from build123d import *

# Parameters (mm, degrees)
SKETCH1_W           = 68
SKETCH1_H           = 33
SKETCH1_R           = 0.95
SKETCH1_W_2         = 52
SKETCH1_H_2         = 17
BOSS_EXTRUDE1_DEPTH = 2
SKETCH2_R           = 4
SKETCH2_R_2         = 0.95
BOSS_EXTRUDE2_DEPTH = 6
FILLET1_R           = 5


with BuildPart() as part:
    # Sketch1 → Boss-Extrude1 (new body)
    with BuildSketch(Plane.XY):
        Rectangle(SKETCH1_W, SKETCH1_H)
        with Locations((-29, 11.5)):
            Circle(SKETCH1_R, mode=Mode.SUBTRACT)
        with Locations((29, 11.5)):
            Circle(SKETCH1_R, mode=Mode.SUBTRACT)
        with Locations((29, -11.5)):
            Circle(SKETCH1_R, mode=Mode.SUBTRACT)
        with Locations((-29, -11.5)):
            Circle(SKETCH1_R, mode=Mode.SUBTRACT)
        Rectangle(SKETCH1_W_2, SKETCH1_H_2, mode=Mode.SUBTRACT)
    extrude(amount=BOSS_EXTRUDE1_DEPTH)

    # Sketch2 → Boss-Extrude2 (add)
    # profile 1 of 4: a face of its own
    with BuildSketch(Plane.XY.offset(2)):
        with Locations(Location((-29, 11.5, 0), (0, 0, 180))):
            Circle(SKETCH2_R)
        with Locations((-29, 11.5)):
            Circle(SKETCH2_R_2, mode=Mode.SUBTRACT)
    # profile 2 of 4: a face of its own
    with BuildSketch(Plane.XY.offset(2)):
        with Locations(Location((29, 11.5, 0), (0, 0, 180))):
            Circle(SKETCH2_R)
        with Locations((29, 11.5)):
            Circle(SKETCH2_R_2, mode=Mode.SUBTRACT)
    # profile 3 of 4: a face of its own
    with BuildSketch(Plane.XY.offset(2)):
        with Locations(Location((29, -11.5, 0), (0, 0, 180))):
            Circle(SKETCH2_R)
        with Locations((29, -11.5)):
            Circle(SKETCH2_R_2, mode=Mode.SUBTRACT)
    # profile 4 of 4: a face of its own
    with BuildSketch(Plane.XY.offset(2)):
        with Locations(Location((-29, -11.5, 0), (0, 0, 180))):
            Circle(SKETCH2_R)
        with Locations((-29, -11.5)):
            Circle(SKETCH2_R_2, mode=Mode.SUBTRACT)
    extrude(amount=BOSS_EXTRUDE2_DEPTH)

    # Fillet1
    fillet1_edges = [part.edges().sort_by_distance(p)[0] for p in [
        (26, -8.5, 1),
        (26, 8.5, 1),
        (-26, 8.5, 1),
        (-26, -8.5, 1),
        (34, -16.5, 1),
        (-34, -16.5, 1),
        (-34, 16.5, 1),
        (34, 16.5, 1),
    ]]
    fillet(fillet1_edges, radius=FILLET1_R)


solid = part.part
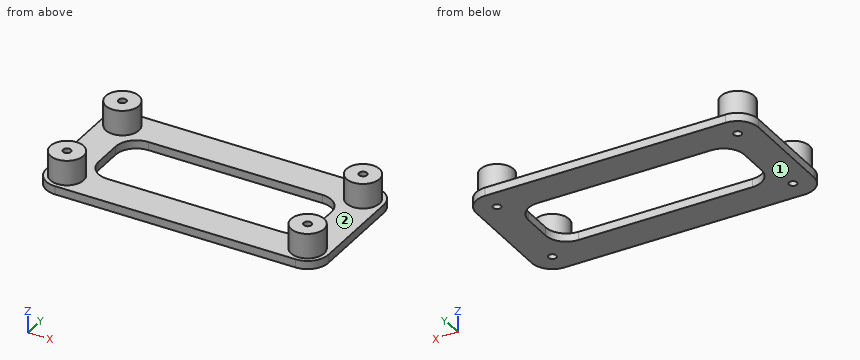
Geometry check sheet. Reference: the model listing, model coordinates, mm. Face numbers are marked on the shaded views. Give positions to 0.01 mm unless a question says otherwise; leave off trailing zeros. Write each loop counter-clockwise with the first axis right and the second up, starting at its lowest first coordinate (ties: lowest second). Pieces come first, ordered by that corner, then holes. Notation, with made-up numbers: M 53.25,-39 L 67.25,-39 A27 ccw 67.25,-22 Z; hole C 80,-24.5 d6. An arc over 180 degrees is marked long. One line per question, with ' | ' between items.
1. Cross-section at A-A (z = 6.25). Enter the section's corners in (x, y), plus the area to 3 significant figures.
Ans:
outline: C -29,-11.5 d8; C -29,11.5 d8; C 29,-11.5 d8; C 29,11.5 d8; hole C -29,-11.5 d1.9; hole C -29,11.5 d1.9; hole C 29,-11.5 d1.9; hole C 29,11.5 d1.9 | area: 190 mm2
2. Mould release check, pull along X, two halves, no side actions. Record for the marked faces 1 and 2: released by +X, released by -X, zero draft, split by the parting line, or undercut.
Ans:
face 1: zero draft | face 2: undercut
3. Scan lines: line 1 along Y through (x, z) = (-29, 2.5); line 2 along Y through (x, z) = (-29, 1.5); line 3 along Y through (x, z) = (17, 0.5). Record each from-to range of solid material in increasing order. Write a range as from..to.
Ans:
line 1: -15.5..-12.45, -10.55..-7.5, 7.5..10.55, 12.45..15.5 | line 2: -16.5..-12.45, -10.55..10.55, 12.45..16.5 | line 3: -16.5..-8.5, 8.5..16.5
4. Cross-section at B-B (y = 0). Enter the section's corners in (x, z), plus the area to 3 significant figures.
Ans:
outline: M -34,0 L -26,0 L -26,2 L -34,2 Z; M 26,0 L 34,0 L 34,2 L 26,2 Z | area: 32.0 mm2
5. Cross-section at C-C (x = 17). Enter the section's corners in (y, z), plus the area to 3 significant figures.
Ans:
outline: M -16.5,0 L -8.5,0 L -8.5,2 L -16.5,2 Z; M 8.5,0 L 16.5,0 L 16.5,2 L 8.5,2 Z | area: 32.0 mm2
